from build123d import *

# Parameters (mm, degrees)
F1_DEPTH = 25.4
F2_W     = 12.7
F2_H     = 12.7
F3_DEPTH = 6.35


with BuildPart() as f1:
    # F0 (on Top) → F1 (new body)
    with BuildSketch(Plane.XY):
        Polygon((0, 25.4), (0, 0), (12.7, 0), (12.7, 12.7), (38.1, 12.7), (38.1, 25.4), align=None)
    extrude(amount=F1_DEPTH)

    # F2 (on face) → F3 (join)
    with BuildSketch(Plane.XZ.offset(-12.7)):
        with Locations((31.75, 6.35)):
            Rectangle(F2_W, F2_H)
    extrude(amount=F3_DEPTH)


solid = f1.part
Input: part model. Units: mm. Frame: model coordinates. A direction names the side the tool comes from. Coordinates: 2 decimals unless noted, no trailing zeros. Loops run counter-clockwise (first coordinate to the right, second up) from the corner with the lowest first, then second, coordinate; pieces in that order, holes last. Notation, with made-up numbers: (50.5, -7) -> (93.5, -7) arc R20 cw to (93.5, 30) -> close; hole circle Ø3 at (28.5, 70). An arc over 180 degrees is marked (long way). Write item = value, one per line. Start each with the question number.
Item 1: Cut plane B-B, the plane x = 27.5. Return loops of the section in (y, z).
Item 2: Cut plane C-C, the plane z = 7. Return loops of the section in (x, y).
Item 3: Reachability of faces 1 (the face through (0, 13, 13)), 2 (the face through (32, 6.35, 6)) from +Z, -Z, +X, -X, +Y, -Y: full face, straight path, thin tool, end or side. Return the list, or none.
Item 4: Material intervals for line 1 (X direction, y = 10, z = 2.5); line 2 (Y direction, x = 16.5, z = 6.5); line 3 (X direction, y = 11.5, z = 21), sorted ascending.
Item 5: First-contact query: P1, Ø6.5, axis at x = 33.5, z = 6.5, coming from the -Y side; P2, Ø7, axis at x = 32, y = 10.5, coming from the +Z side; P3, Ø6, axis at x = 32.5, y = 3, coming from the -Z side; P4, Ø1, axis at y = 2.5, z = 7, coming from the +X side. Flat tips, straight axial feed; report the tip coordinate or a pass-through.
Item 6: Cut plane D-D, the plane y = 1.5. Return loops of the section in (x, z).
Item 7: Cut plane A-A, the plane y = 9. Return loops of the section in (x, z).
Item 8: Mould query, pull axis X, two halves, no side actions, for faces 3 (the face through (32, 10, 12.7)), 4 (the face through (38.1, 18, 13)), 5 (the face through (12.7, 6, 13)), 6 (the face through (25.4, 10, 6)). Classes: pulls with the +X half, pulls with the -X half, needs draft (parallel to the pull), parting line crosses it, or undercut.
Ans:
q1.outline = (6.35, 0) -> (25.4, 0) -> (25.4, 25.4) -> (12.7, 25.4) -> (12.7, 12.7) -> (6.35, 12.7) -> close
q2.outline = (0, 0) -> (12.7, 0) -> (12.7, 12.7) -> (25.4, 12.7) -> (25.4, 6.35) -> (38.1, 6.35) -> (38.1, 25.4) -> (0, 25.4) -> close
q3.face_1 = +Z, -Z, -X, +Y, -Y
q3.face_2 = +Z, -Z, +X, -Y
q4.line_1 = 0 to 12.7, 25.4 to 38.1
q4.line_2 = 12.7 to 25.4
q4.line_3 = 0 to 12.7
q5.P1 = 6.35
q5.P2 = 25.4
q5.P3 = through
q5.P4 = 12.7
q6.outline = (0, 0) -> (12.7, 0) -> (12.7, 25.4) -> (0, 25.4) -> close
q7.outline = (0, 0) -> (12.7, 0) -> (12.7, 25.4) -> (0, 25.4) -> close; (25.4, 0) -> (38.1, 0) -> (38.1, 12.7) -> (25.4, 12.7) -> close
q8.face_3 = needs draft
q8.face_4 = pulls with the +X half
q8.face_5 = undercut
q8.face_6 = undercut
